from build123d import *

# Parameters (mm, degrees)
SKETCH_1_W      = 60
SKETCH_1_H      = 40
EXTRUDE_1_DEPTH = 130
CHAMFER_1_SIZE  = 10


with BuildPart() as part:
    # 草图1 → 凸台-拉伸1 (new body)
    with BuildSketch(Plane.XY):
        with Locations((30, -20)):
            Rectangle(SKETCH_1_W, SKETCH_1_H)
    extrude(amount=EXTRUDE_1_DEPTH)

    # 倒角1
    chamfer_1_edges = [part.edges().sort_by_distance(p)[0] for p in [
        (60, 0, 65),
        (0, -40, 65),
    ]]
    chamfer(chamfer_1_edges, length=CHAMFER_1_SIZE)


solid = part.part
Input: part model. Units: mm. Frame: model coordinates. Give positions to 0.01 mm unless a question says otherwise; leave off trailing zeros. Write each loop counter-clockwise with the first axis right and the second up, starting at its lowest first coordinate (ties: lowest second). Pieces come first, ordered by that corner, then holes. Notation, with made-up numbers: (71, -5.75) -> (92, -5.75) arc R19 cw to (92, 5.25) -> close; hole circle Ø2 at (74, 31.25). An arc over 180 degrees is marked (long way). Use one line per item in the form item = value. Start each with the question number.
1) Ray query, probe 1 along X at (y, z) = (-5.5, 98); probe 2 along X at (y, z) = (-3.5, 99.5); probe 3 along Y at (x, z) = (6, 67.5). Return the intervals inside material, ascending. Write a range as from..to.
2) Section query C-C on x = 5.5. Return the cut outline in (y, z).
3) Section query A-A on z = 48.5. Return the cut outline in (x, y), then the cut area to 3 significant figures.
4) Section query B-B on x = 53.5. Return the cut outline in (y, z).
Outcome:
q1.probe_1 = 0..55.5
q1.probe_2 = 0..53.5
q1.probe_3 = -36..0
q2.outline = (-35.5, 0) -> (0, 0) -> (0, 130) -> (-35.5, 130) -> close
q3.outline = (0, -30) -> (10, -40) -> (60, -40) -> (60, -10) -> (50, 0) -> (0, 0) -> close
q3.area = 2,300 mm^2
q4.outline = (-40, 0) -> (-3.5, 0) -> (-3.5, 130) -> (-40, 130) -> close
